Geometry: final body of the model. Coordinates: model frame, mm. Face numbers are marked on the shaded views. A direction names the side the tool comes from. Give positions to 0.01 mm unless a question says otherwise; leave off trailing zeros. Order: outer loops, then holes, each group sorted by start corner. A loop starts at its lowest first (then second) coordinate and runs counter-clockwise, first axis right, second up. Notation, with made-up numbers: M 1.25,-31 L 15.25,-31 A13 cw 15.25,-16 Z; hole C 69.25,56.5 d7. An arc over 180 degrees is marked long. Write item = value, one per line. Start each with the question number.
from build123d import *

# Parameters (mm, degrees)
SKETCH2_W           = 90
SKETCH2_H           = 78
BOSS_EXTRUDE1_DEPTH = 8
SKETCH3_R           = 12.5
SKETCH3_R_2         = 7.5
BOSS_EXTRUDE2_DEPTH = 50
BOSS_EXTRUDE3_DEPTH = 8
FILLET1_R           = 15
FILLET2_R           = 15


with BuildPart() as part:
    # Sketch2 → Boss-Extrude1 (new body)
    with BuildSketch(Plane(origin=(0, 0, 0), x_dir=(1, 0, 0), z_dir=(0, 1, 0))):
        with Locations((45, 39)):
            Rectangle(SKETCH2_W, SKETCH2_H)
    extrude(amount=BOSS_EXTRUDE1_DEPTH)



with BuildPart() as body_2:
    # Sketch3 → Boss-Extrude2 (new body)
    with BuildSketch(Plane(origin=(90, 0, 0), x_dir=(0, 0, -1), z_dir=(1, 0, 0))):
        with Locations((33, 67)):
            Circle(SKETCH3_R)
        with Locations((33, 67)):
            Circle(SKETCH3_R_2, mode=Mode.SUBTRACT)
    extrude(amount=-BOSS_EXTRUDE2_DEPTH)


with BuildPart() as part_1:
    add(part.part)

    add(body_2.part)  # Boss-Extrude3 merges body 2
    # Sketch4 → Boss-Extrude3 (add)
    with BuildSketch(Plane(origin=(90, 0, 0), x_dir=(0, 0, -1), z_dir=(1, 0, 0))):
        with BuildLine():
            Line((44.074003649, 72.797968885), (78, 8))
            Line((78, 8), (0, 8))
            Line((0, 8), (21.150362392, 70.979458323))
            ThreePointArc((21.150362392, 70.979458323), (33.988507549, 54.539147187), (44.074003649, 72.797968885))
        make_face()
    extrude(amount=-BOSS_EXTRUDE3_DEPTH)

    # Fillet1
    fillet1_edges = [part_1.edges().sort_by_distance(p)[0] for p in [
        (0, 4, 0),
    ]]
    fillet(fillet1_edges, radius=FILLET1_R)

    # Fillet2
    fillet2_edges = [part_1.edges().sort_by_distance(p)[0] for p in [
        (0, 4, -78),
    ]]
    fillet(fillet2_edges, radius=FILLET2_R)


solid = part_1.part
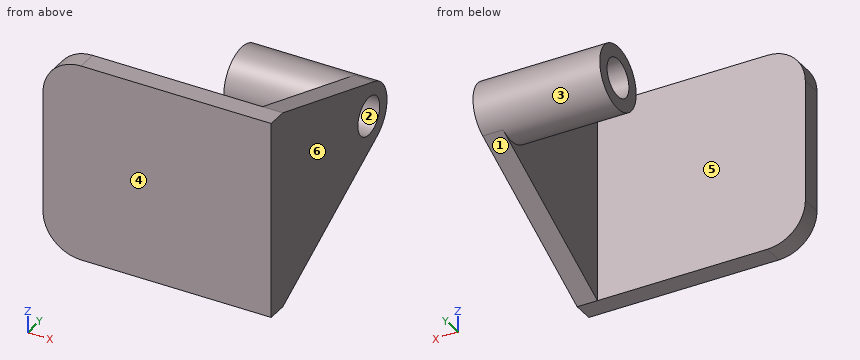
1) Cut plane C-C (y = 67). Return loops of the section in (x, z), plus the area to 3 significant figures.
2) Draft query along Z for the marked faces 1, 2, 3 and 4. Return one class per face: pulls with the +Z half, pulls with the -Z half, needs draft (parallel to the pull), parting line crosses it, or undercut.
3) Cut plane A-A (x = 59). Return loops of the section in (y, z).
4) Cut plane D-D (z = -52.5). Return loops of the section in (x, y).
5) Cut plane B-B (z = -33). Return loops of the section in (x, y), plus the area to 3 significant figures.
6) Access query for the marked faces 5 and 6. Directions: +Z, -Z, +X, -X, +Y, -Y. A direction counts if a zero-diameter tool reaches every point of the face in a straight line with its end or side. Return the directions, or none.
7) Ray query, L1, parallel to Y at x = 54, z = -33; L2, parallel to X at y = 10.5, z = -24.5; L3, parallel to X at y = 71, z = -26. Return the intervals inside material, ascending.
8) Pin query (flat end, axial travel): pin 1 Ø5 at (x, z) = (21, -8.5) entering from +Y; pin 2 Ø20 at (y, z) = (66, -27) entering from -X; pin 3 Ø8 at (y, z) = (20, -26) entering from -X. Return the tip coordinate at first contact, or that it passes through.
Reply:
q1.outline = M 40,-45.5 L 82,-45.5 L 82,-47.11 L 90,-47.11 L 90,-40.5 L 40,-40.5 Z; M 40,-25.5 L 90,-25.5 L 90,-19.81 L 82,-19.81 L 82,-20.5 L 40,-20.5 Z
q1.area = 518 mm²
q2.face_1 = pulls with the -Z half
q2.face_2 = undercut
q2.face_3 = parting line crosses it
q2.face_4 = needs draft
q3.outline = M 0,-78 L 8,-78 L 8,0 L 0,0 Z; C 67,-33 d25; hole C 67,-33 d15
q4.outline = M 0,0 L 90,0 L 90,56.7 L 82,56.7 L 82,8 L 0,8 Z
q5.outline = M 0,0 L 90,0 L 90,59.5 L 40,59.5 L 40,54.5 L 82,54.5 L 82,8 L 0,8 Z; M 40,74.5 L 90,74.5 L 90,79.5 L 40,79.5 Z
q5.area = 1,590 mm²
q6.face_5 = +Z, -Z, -X
q6.face_6 = +Z, -Z, +X, +Y, -Y
q7.L1 = 0 to 8, 54.5 to 59.5, 74.5 to 79.5
q7.L2 = 82 to 90
q7.L3 = 40 to 90
q8.pin_1 = 8
q8.pin_2 = 40
q8.pin_3 = 82
